Answer from the drawing. Dimensions are ordinates in mm from the lowest x, y and z of the part. Round coordinates to 2 decimals unless told otherwise and drop trailing zeros. Loops run counter-clockwise (first coordinate to the right, second up) from the corner with the lowest first, then second, coordinate; pieces in that order, holes last. Notation, with made-up numbers: (21.5, 59) - (72.5, 59) arc R6 ccw to (72.5, 68) - close; hole circle Ø3 at (-8.5, 66). An arc over 180 degrees is marked (long way). Answer as CSV lines item,"result". Start each with the question number.
Q1. Section D-D on y = 0.4 is taken. Count the separate pieces of the cut face and the enclosed holes in it, then the cut area to 3 significant figures.
Q2. Section B-B on x = 1.27 is taken. Write down the section's boundary in (y, z).
Q3. Straight lines are drawn through the part: L1, parallel to X at y = 1.1, z = 3.81; L2, parallel to X at y = 1.1, z = 1.27; L3, parallel to X at y = 1.35, z = 3.5. For each, find the intervals that lie inside material, in ascending order. Write a range as [from, to].
Q4. Section C-C on z = 1.27 is taken. Write down the section's boundary in (x, y).
Q5. Section A-A on z = 16.51 is taken. Write down the section's boundary in (x, y).
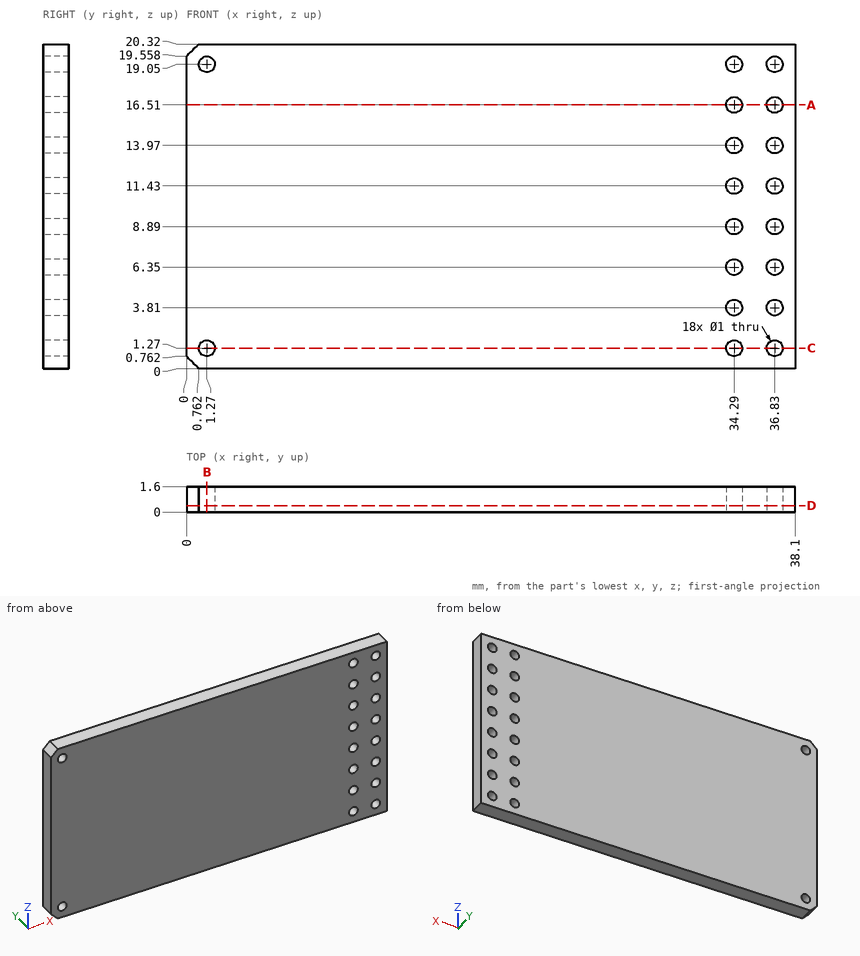
Findings:
1,separate pieces,"1"
1,enclosed holes,"18"
1,area,"759 mm^2"
2,outline,"(0, 0) - (1.6, 0) - (1.6, 0.77) - (0, 0.77) - close; (0, 1.77) - (1.6, 1.77) - (1.6, 18.55) - (0, 18.55) - close; (0, 19.55) - (1.6, 19.55) - (1.6, 20.32) - (0, 20.32) - close"
3,L1,"x = [0, 33.79], [34.79, 36.33], [37.33, 38.1]"
3,L2,"x = [0, 0.77], [1.77, 33.79], [34.79, 36.33], [37.33, 38.1]"
3,L3,"x = [0, 33.9], [34.68, 36.44], [37.22, 38.1]"
4,outline,"(0, 0) - (0.77, 0) - (0.77, 1.6) - (0, 1.6) - close; (1.77, 0) - (33.79, 0) - (33.79, 1.6) - (1.77, 1.6) - close; (34.79, 0) - (36.33, 0) - (36.33, 1.6) - (34.79, 1.6) - close; (37.33, 0) - (38.1, 0) - (38.1, 1.6) - (37.33, 1.6) - close"
5,outline,"(0, 0) - (33.79, 0) - (33.79, 1.6) - (0, 1.6) - close; (34.79, 0) - (36.33, 0) - (36.33, 1.6) - (34.79, 1.6) - close; (37.33, 0) - (38.1, 0) - (38.1, 1.6) - (37.33, 1.6) - close"
